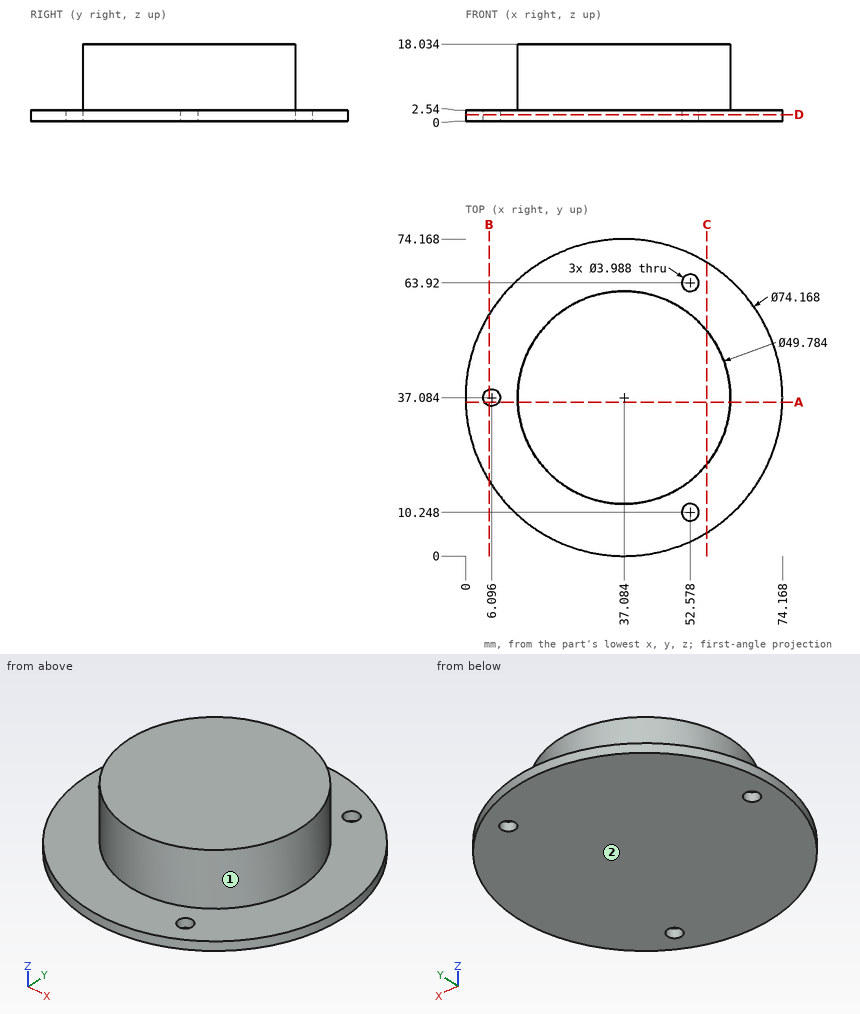
The figure shows three views and two pictorial views of one solid part (mm, origin at its lowest corner). Answer the questions. A direction names the side the tool comes from. Give positions to 0.01 mm unless a question says otherwise; leave off trailing zeros. Loops run counter-clockwise (first coordinate to the right, second up) from the corner with the lowest first, then second, coordinate; pieces in that order, holes last. Notation, with made-up numbers: (-27, 25.5) -> (11, 25.5) arc R14 ccw to (11, 41.5) -> close; hole circle Ø3 at (52.5, -1). An arc over 180 degrees is marked (long way). Put each result on its own line as item: value. Start each with the question number.
Item 1: Find the intervals of material crossed by L1, parallel to Z at x = 49, y = 59.5; L2, parallel to Y at x = 38.5, z = 10.5 (1 decimal); L3, parallel to Y at x = 34.5, z = 11.75, in increasing order. Write a range as [from, to].
Item 2: The part is cut by section B-B (x = 5.5). Give the vertices of the cut face in (y, z).
Item 3: Each of these flat-tipped pins is pushed along its axis until it touches: P1, Ø1.5, axis at x = 54, z = 11, coming from the -Y side (1 decimal); P2, Ø4, axis at y = 16.5, z = 8.5, coming from the -X side (1 decimal); P3, Ø5, axis at x = 52.58, y = 63.92, coming from the +Z side. Where does it stop, or does it pass through?
Item 4: The part is cut by section D-D (z = 1.5). Give the vertices of the cut face in (x, y), then the cut area to 3 significant figures.
Item 5: Which of the six approach directions +Z, -Z, +X, -X, +Y, -Y give full straight-line access (tool end or side, diameter ignored) to the marked faces 1 and 2?
Item 6: The part is cut by section A-A (y = 36). Give the vertices of the cut face in (x, z) (1 decimal).
Item 7: The part is cut by section C-C (x = 56.5). Give the vertices of the cut face in (y, z), then the cut area to 3 significant figures.
Answers below:
1. L1: [0, 2.54]
1. L2: [12.2, 61.9]
1. L3: [12.33, 61.84]
2. outline: (17.65, 0) -> (35.18, 0) -> (35.18, 2.54) -> (17.65, 2.54) -> close; (38.99, 0) -> (56.52, 0) -> (56.52, 2.54) -> (38.99, 2.54) -> close
3. P1: y = 18.2
3. P2: x = 20.5
3. P3: z = 2.54
4. outline: circle Ø74.17 at (37.08, 37.08); hole circle Ø3.99 at (6.1, 37.08); hole circle Ø3.99 at (52.58, 10.25); hole circle Ø3.99 at (52.58, 63.92)
4. area: 4,280 mm2
5. face 1: +Z
5. face 2: -Z, +X, -X, +Y, -Y
6. outline: (0, 0) -> (4.4, 0) -> (4.4, 2.5) -> (0, 2.5) -> close; (7.8, 0) -> (74.2, 0) -> (74.2, 2.5) -> (62, 2.5) -> (62, 18) -> (12.2, 18) -> (12.2, 2.5) -> (7.8, 2.5) -> close
7. outline: (5.49, 0) -> (68.68, 0) -> (68.68, 2.54) -> (52.66, 2.54) -> (52.66, 18.03) -> (21.51, 18.03) -> (21.51, 2.54) -> (5.49, 2.54) -> close
7. area: 643 mm2
